Can you work these out from the model? Positions are in its coordinate system, mm. A direction names the side the tool comes from. Round coordinates to 2 decimals unless told otherwise and drop trailing zeros. Write each loop counter-clockwise with the first axis right and the second up, starting at its lowest first coordinate (ties: lowest second). Pieces come first, ordered by that corner, then holes. Notation, with made-up numbers: (63.25, -23.75) -> (111.25, -23.75) arc R22 ccw to (111.25, 5.25) -> close; hole circle Ø9 at (60, 49). An arc over 180 degrees is marked (long way). Write item = value, one per line. Start each with the question number.
1) Imagine slicing it at A-A, the plane x = 23.5. Please give me the cut outline in (y, z), then the cut area to 3 significant figures.
2) If I drill on line 1 (Z direction, x = 103.5, y = -10.5); line 2 (Z direction, x = 24.5, y = 43.5); line 3 (Z direction, x = 61, y = 36), over which ranges is the centre line in solid material (lowest first)?
3) Imagine slicing it at C-C, the plane z = -43. Please give me the cut outline in (x, y).
4) Imagine slicing it at B-B, the plane y = 15. Please give me the cut outline in (x, z).
5) I'm going to push flat-ended pins straight in: pin 1 (3 mm diameter, centred on y = -7, z = -3, fed in from +X); pin 2 (16.5 mm diameter, centred on x = 89.5, y = -8.5, fed in from +Z); pin 3 (12 mm diameter, centred on x = 30.5, y = -5, fed in from +Z); pin 4 (1 mm diameter, centred on x = 56, z = -42.5, fed in from -Y). Where does each tip first touch, or does it pass through?
6) Thinking about a two-plate mould opening in Z: for faces 1 (the face through (63, 45, -29)), 2 (the face through (63, 40, -51)), 3 (the face through (63, 38, -43)), 4 (the face through (31, -7, -2)), which applies, +Z half, -Z half, draft (parallel to the pull), parting line (faces both ways), or undercut?
7) For faces 5 (the face through (21.25, -7, -4)), 6 (the face through (63, 35, -48)), 7 (the face through (41.25, -7, -4)), which set-ups out of +Z, -Z, +X, -X, +Y, -Y let a thin tool reach every point of the face, with its end or its side?
from build123d import *

# Parameters (mm, degrees)
SKETCH_1_W      = 125
SKETCH_1_H      = 8
EXTRUDE_1_DEPTH = 60
SKETCH_2_W      = 50
SKETCH_2_H      = 10
EXTRUDE_2_DEPTH = 43
SKETCH_3_W      = 20
SKETCH_3_H      = 4
EXTRUDE_3_DEPTH = 15
SKETCH_4_W      = 50
SKETCH_4_H      = 3


with BuildPart() as part:
    # 草图1 → 凸台-拉伸1 (new body)
    with BuildSketch(Plane(origin=(0, 0, 0), x_dir=(1, 0, 0), z_dir=(0, 1, 0))):
        with Locations((62.5, 4)):
            Rectangle(SKETCH_1_W, SKETCH_1_H)
    extrude(amount=EXTRUDE_1_DEPTH)

    # 草图2 → 凸台-拉伸2 (add)
    with BuildSketch(Plane(origin=(0, 0, -8), x_dir=(-1, 0, 0), z_dir=(0, 0, -1))):
        with Locations((-62.5, 40)):
            Rectangle(SKETCH_2_W, SKETCH_2_H)
    extrude(amount=EXTRUDE_2_DEPTH)

    # 草图3 → 凸台-拉伸3 (add)
    with BuildSketch(Plane.XZ):
        with Locations((31.25, -4)):
            Rectangle(SKETCH_3_W, SKETCH_3_H)
        with Locations((93.75, -4)):
            Rectangle(SKETCH_3_W, SKETCH_3_H)
    extrude(amount=EXTRUDE_3_DEPTH)

    # 草图4 → 切除-旋转1 (revolve, cut)
    with BuildSketch(Plane.XZ.offset(-35)):
        with Locations((62.5, -44.5)):
            Rectangle(SKETCH_4_W, SKETCH_4_H)
    revolve(axis=Axis((37.5, 35, -43), (1, 0, 0)), mode=Mode.SUBTRACT)


solid = part.part
Reported:
q1.outline = (-15, -6) -> (0, -6) -> (0, -8) -> (60, -8) -> (60, 0) -> (0, 0) -> (0, -2) -> (-15, -2) -> close
q1.area = 540 mm²
q2.line_1 = -6 to -2
q2.line_2 = -8 to 0
q2.line_3 = -51 to -45.83, -40.17 to 0
q3.outline = (37.5, 38) -> (87.5, 38) -> (87.5, 45) -> (37.5, 45) -> close
q4.outline = (0, -8) -> (125, -8) -> (125, 0) -> (0, 0) -> close
q5.pin_1 = 103.75
q5.pin_2 = -2
q5.pin_3 = 0
q5.pin_4 = 37.83
q6.face_1 = draft
q6.face_2 = -Z half
q6.face_3 = undercut
q6.face_4 = +Z half
q7.face_5 = +Z, -Z, -X, -Y
q7.face_6 = -Z, +X, -X, -Y
q7.face_7 = +Z, -Z, -Y
